Can you work these out from the drawing? Everything is in mm from the part's minimum corner. Give positions to 0.01 mm unless a question says otherwise; leave off trailing zeros. Order: outer loops, then holes, each group sorted by start corner. A loop starts at its lowest first (then second) coordinate and runs counter-clockwise, first axis right, second up. Notation, with made-up numbers: (14.5, 31.25) -> (55.5, 31.25) arc R26 cw to (55.5, 67.25) -> close; hole circle Ø10 at (-5, 61). An arc over 180 degrees is marked (long way). One line per item, written item: value.
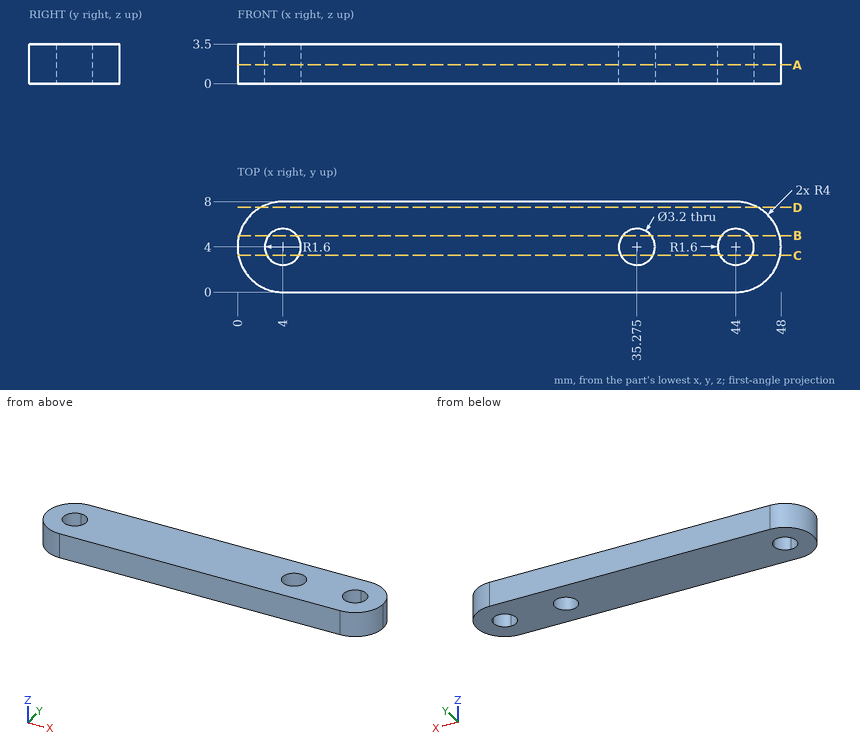
1) Suppose I cut it at A-A, the plane z = 1.65. Write out the boundary of the cut face in (x, y) (1 decimal).
Answer below:
outline: (4, 0) -> (44, 0) arc R4 ccw to (44, 8) -> (4, 8) arc R4 ccw to start; hole circle Ø3.2 at (4, 4); hole circle Ø3.2 at (35.3, 4); hole circle Ø3.2 at (44, 4)
2) Suppose I cut it at C-C, the plane y = 3.25. Write out the boundary of the cut face in (x, z), then the cut area to 3 significant figures.
Answer below:
outline: (0.07, 0) -> (2.59, 0) -> (2.59, 3.5) -> (0.07, 3.5) -> close; (5.41, 0) -> (33.86, 0) -> (33.86, 3.5) -> (5.41, 3.5) -> close; (36.69, 0) -> (42.59, 0) -> (42.59, 3.5) -> (36.69, 3.5) -> close; (45.41, 0) -> (47.93, 0) -> (47.93, 3.5) -> (45.41, 3.5) -> close
area: 138 mm2
3) Suppose I cut it at B-B, the plane y = 5. Write out the boundary of the cut face in (x, z).
Answer below:
outline: (0.13, 0) -> (2.75, 0) -> (2.75, 3.5) -> (0.13, 3.5) -> close; (5.25, 0) -> (34.03, 0) -> (34.03, 3.5) -> (5.25, 3.5) -> close; (36.52, 0) -> (42.75, 0) -> (42.75, 3.5) -> (36.52, 3.5) -> close; (45.25, 0) -> (47.87, 0) -> (47.87, 3.5) -> (45.25, 3.5) -> close
4) If I drill on line 1 along X through (y, z) = (4.75, 0.65); line 2 along Y through (x, z) = (5, 1.75); line 3 along Y through (x, z) = (34, 1.3) (1 decimal), over which ranges is the centre line in solid material (lowest first)?
Answer below:
line 1: x = 0.07 to 2.59, 5.41 to 33.86, 36.69 to 42.59, 45.41 to 47.93
line 2: y = 0 to 2.75, 5.25 to 8
line 3: y = 0 to 3, 5 to 8
5) Suppose I cut it at D-D, the plane y = 7.5. Write out the boundary of the cut face in (x, z), then the cut area to 3 significant figures.
Answer below:
outline: (2.06, 0) -> (45.94, 0) -> (45.94, 3.5) -> (2.06, 3.5) -> close
area: 154 mm2
